Verification items for the finished model (mm, model axes). Round coordinates to 2 decimals unless told otherwise and drop trailing zeros. Answer as a JSON object with one key per item and string values.
```python
from build123d import *

# Parameters (mm, degrees)
SKETCH1_W           = 12
SKETCH1_H           = 12
SKETCH1_R           = 2.5
SKETCH1_W_2         = 71
SKETCH1_H_2         = 24
SKETCH1_R_2         = 5
BOSS_EXTRUDE1_DEPTH = 3


with BuildPart() as part:
    # Sketch1 → Boss-Extrude1 (new body)
    with BuildSketch(Plane(origin=(0, 0, 0), x_dir=(1, 0, 0), z_dir=(0, 1, 0))):
        Polygon((-28, -20), (33.6, -20), (33.6, -17), (98.2, -17), (98.2, -20), (162.8, -20), (162.8, -17), (227.4, -17), (227.4, -20), (289, -20), (289, 99.936143656), (227.417055149, 100), (227.417055149, 97), (162.817055149, 97), (162.817055149, 100), (98.2, 100), (98.2, 97), (33.6, 97), (33.6, 100), (-28, 100), align=None)
        with Locations((6, 6)):
            Rectangle(SKETCH1_W, SKETCH1_H, mode=Mode.SUBTRACT)
        with Locations((23, 6)):
            Rectangle(SKETCH1_W, SKETCH1_H, mode=Mode.SUBTRACT)
        with Locations((40, 6)):
            Rectangle(SKETCH1_W, SKETCH1_H, mode=Mode.SUBTRACT)
        with Locations((57, 6)):
            Rectangle(SKETCH1_W, SKETCH1_H, mode=Mode.SUBTRACT)
        with Locations((74, 6)):
            Rectangle(SKETCH1_W, SKETCH1_H, mode=Mode.SUBTRACT)
        with Locations((91, 6)):
            Rectangle(SKETCH1_W, SKETCH1_H, mode=Mode.SUBTRACT)
        with Locations((108, 6)):
            Rectangle(SKETCH1_W, SKETCH1_H, mode=Mode.SUBTRACT)
        with Locations((125, 6)):
            Rectangle(SKETCH1_W, SKETCH1_H, mode=Mode.SUBTRACT)
        with Locations(Location((6.5, 17.5, 0), (0, 0, 270))):
            Circle(SKETCH1_R, mode=Mode.SUBTRACT)
        with Locations(Location((23.5, 17.5, 0), (0, 0, 270))):
            Circle(SKETCH1_R, mode=Mode.SUBTRACT)
        with Locations(Location((40.5, 17.5, 0), (0, 0, 270))):
            Circle(SKETCH1_R, mode=Mode.SUBTRACT)
        with Locations((31, 35)):
            Rectangle(SKETCH1_W, SKETCH1_H, mode=Mode.SUBTRACT)
        with Locations(Location((57.5, 17.5, 0), (0, 0, 270))):
            Circle(SKETCH1_R, mode=Mode.SUBTRACT)
        with Locations(Location((74.5, 17.5, 0), (0, 0, 270))):
            Circle(SKETCH1_R, mode=Mode.SUBTRACT)
        with Locations(Location((91.5, 17.5, 0), (0, 0, 270))):
            Circle(SKETCH1_R, mode=Mode.SUBTRACT)
        with Locations(Location((108.5, 17.5, 0), (0, 0, 270))):
            Circle(SKETCH1_R, mode=Mode.SUBTRACT)
        with Locations(Location((125.5, 17.5, 0), (0, 0, 270))):
            Circle(SKETCH1_R, mode=Mode.SUBTRACT)
        with Locations((54, 35)):
            Rectangle(SKETCH1_W, SKETCH1_H, mode=Mode.SUBTRACT)
        with Locations((77, 35)):
            Rectangle(SKETCH1_W, SKETCH1_H, mode=Mode.SUBTRACT)
        with Locations((142, 6)):
            Rectangle(SKETCH1_W, SKETCH1_H, mode=Mode.SUBTRACT)
        with Locations((159, 6)):
            Rectangle(SKETCH1_W, SKETCH1_H, mode=Mode.SUBTRACT)
        with Locations((176, 6)):
            Rectangle(SKETCH1_W, SKETCH1_H, mode=Mode.SUBTRACT)
        with Locations((193, 6)):
            Rectangle(SKETCH1_W, SKETCH1_H, mode=Mode.SUBTRACT)
        with Locations((210, 6)):
            Rectangle(SKETCH1_W, SKETCH1_H, mode=Mode.SUBTRACT)
        with Locations((227, 6)):
            Rectangle(SKETCH1_W, SKETCH1_H, mode=Mode.SUBTRACT)
        with Locations((244, 6)):
            Rectangle(SKETCH1_W, SKETCH1_H, mode=Mode.SUBTRACT)
        with Locations((261, 6)):
            Rectangle(SKETCH1_W, SKETCH1_H, mode=Mode.SUBTRACT)
        with Locations(Location((142.5, 17.5, 0), (0, 0, 270))):
            Circle(SKETCH1_R, mode=Mode.SUBTRACT)
        with Locations(Location((159.5, 17.5, 0), (0, 0, 270))):
            Circle(SKETCH1_R, mode=Mode.SUBTRACT)
        with Locations(Location((176.5, 17.5, 0), (0, 0, 270))):
            Circle(SKETCH1_R, mode=Mode.SUBTRACT)
        with Locations(Location((193.5, 17.5, 0), (0, 0, 270))):
            Circle(SKETCH1_R, mode=Mode.SUBTRACT)
        with Locations(Location((210.5, 17.5, 0), (0, 0, 270))):
            Circle(SKETCH1_R, mode=Mode.SUBTRACT)
        with Locations(Location((227.5, 17.5, 0), (0, 0, 270))):
            Circle(SKETCH1_R, mode=Mode.SUBTRACT)
        with Locations(Location((244.5, 17.5, 0), (0, 0, 270))):
            Circle(SKETCH1_R, mode=Mode.SUBTRACT)
        with Locations(Location((261.5, 17.5, 0), (0, 0, 270))):
            Circle(SKETCH1_R, mode=Mode.SUBTRACT)
        with Locations(Location((31.5, 46.5, 0), (0, 0, 270))):
            Circle(SKETCH1_R, mode=Mode.SUBTRACT)
        with Locations(Location((54.5, 46.5, 0), (0, 0, 270))):
            Circle(SKETCH1_R, mode=Mode.SUBTRACT)
        with Locations(Location((77.5, 46.5, 0), (0, 0, 270))):
            Circle(SKETCH1_R, mode=Mode.SUBTRACT)
        with Locations((54.5, 68)):
            Rectangle(SKETCH1_W_2, SKETCH1_H_2, mode=Mode.SUBTRACT)
        with Locations((136, 45)):
            Rectangle(SKETCH1_W, SKETCH1_H, mode=Mode.SUBTRACT)
        with Locations((159, 45)):
            Rectangle(SKETCH1_W, SKETCH1_H, mode=Mode.SUBTRACT)
        with Locations(Location((135.5, 56.5, 0), (0, 0, 270))):
            Circle(SKETCH1_R, mode=Mode.SUBTRACT)
        with Locations(Location((158.5, 56.5, 0), (0, 0, 270))):
            Circle(SKETCH1_R, mode=Mode.SUBTRACT)
        with Locations((211, 45.2)):
            Rectangle(SKETCH1_W, SKETCH1_H, mode=Mode.SUBTRACT)
        with Locations((236, 45.2)):
            Rectangle(SKETCH1_W, SKETCH1_H, mode=Mode.SUBTRACT)
        with Locations(Location((211, 56.7, 0), (0, 0, 270))):
            Circle(SKETCH1_R, mode=Mode.SUBTRACT)
        with Locations(Location((236, 56.7, 0), (0, 0, 270))):
            Circle(SKETCH1_R, mode=Mode.SUBTRACT)
        with Locations(Location((132, 74, 0), (0, 0, 270))):
            Circle(SKETCH1_R_2, mode=Mode.SUBTRACT)
        with Locations(Location((162, 74, 0), (0, 0, 270))):
            Circle(SKETCH1_R_2, mode=Mode.SUBTRACT)
        with Locations((211, 70.2)):
            Rectangle(SKETCH1_W, SKETCH1_H, mode=Mode.SUBTRACT)
        with Locations((236, 70.2)):
            Rectangle(SKETCH1_W, SKETCH1_H, mode=Mode.SUBTRACT)
        with Locations(Location((211, 81.7, 0), (0, 0, 270))):
            Circle(SKETCH1_R, mode=Mode.SUBTRACT)
        with Locations(Location((236, 81.7, 0), (0, 0, 270))):
            Circle(SKETCH1_R, mode=Mode.SUBTRACT)
    extrude(amount=BOSS_EXTRUDE1_DEPTH)


solid = part.part
```
Q1. Gauge pin test, flat end, axial feed: P1, Ø0.9, axis at x = 243.5, y = 1.5, coming from the -Z side. Record the tip position at first contact, or that the pin passes through.
Geometry check:
{"P1": "stops at z = -99.98"}
Q2. Material ranges on line 1 along X through (y, z) = (1, -56.7); line 2 along X through (y, z) = (0.2, -32.5); line 3 along Z through (x, y) = (227.5, 1.5), recorded low to high. Write a range as [from, to].
Geometry check:
{"line 1": "x = [-28, 19], [90, 133.01], [137.99, 156.01], [160.99, 208.5], [213.5, 233.5], [238.5, 289]", "line 2": "x = [-28, 25], [37, 48], [60, 71], [83, 289]", "line 3": "z = [-100, -20], [-15, -12], [0, 20]"}
Q3. Section check A-A, the plane y = 2.3. State how many separate pieces and enclosed holes the cut face has, then the cut area to 3 significant figures.
Geometry check:
{"separate pieces": "1", "enclosed holes": "53", "area": "31,300 mm2"}
Q4. Release check for a two-part mould opening along Z. For faces 1 (the cylindrical face through (130.085, 1.479, -69.381)), 2 (the flat face through (128, 3, -41)) record: released by +Z, released by -Z, zero draft, split by the parting line, or undercut.
Geometry check:
{"face 1": "undercut", "face 2": "zero draft"}
